Autodesk Inventor part; units mm, degrees
ref_plane "YZ Plane" through (0, 0, 0) normal (1, 0, 0) x (0, 1, 0)
ref_plane "XZ Plane" through (0, 0, 0) normal (0, 1, 0) x (-1, 0, 0)
ref_plane "XY Plane" through (0, 0, 0) normal (0, 0, 1) x (1, 0, 0)
sketch "Sketch1" plane through (0, 0, 0) normal (0, 0, 1) x (1, 0, 0)
  arc A0 (12.6748, 0.8001) -> (12.6748, -0.8001) centre (0, 0) ccw
  line L0 (-14.732, 25.4) -> (25.4, 25.4)
  line L1 (8.89, -14.732) -> (-8.382, -14.732)
  line L2 (-14.732, -8.382) -> (-14.732, 25.4)
  line L3 (-14.732, -8.382) -> (-8.382, -14.732)
  line L4 (8.89, -14.732) -> (15.24, -8.382)
  line L5 (15.24, -8.382) -> (25.4, -8.382)
  line L6 (-22.7584, 0) -> (33.4264, 0) construction
  line L7 (0, -22.7584) -> (0, 33.4264) construction
  line L8 (12.6748, 0.8001) -> (25.4, 0.8001)
  line L9 (12.6748, -0.8001) -> (25.4, -0.8001)
  line L10 (25.4, 25.4) -> (25.4, 0.8001)
  line L11 (25.4, -0.8001) -> (25.4, -8.382)
  dimension "d0" = 25.4
  dimension "d1" = 14.732
  dimension "d2" = 14.732
  dimension "d4" = 25.4
  dimension "d9" = 1.6002
  dimension "d11" = 45
  dimension "d12" = 25.4
  dimension "d14" = 8.89
  dimension "d15" = 15.24
  dimension "d49" = 45
extrude "Extrusion1" add sketch "Sketch1" along normal blind 12.7
sketch "Sketch2" plane through (0, 0, 12.7) normal (0, 0, 1) x (1, 0, 0)
  line L0 (-14.732, -8.382) -> (-14.732, 25.4)
  line L1 (-14.732, 25.4) -> (25.4, 25.4)
  line L2 (25.4, 25.4) -> (25.4, 0.8001)
  line L3 (-22.7584, 0) -> (33.4264, 0) construction
  line L4 (0, -22.7584) -> (0, 33.4264) construction
  line L5 (-11.557, 25.4) -> (22.225, 25.4)
  line L6 (22.225, 25.4) -> (22.225, 15.875)
  line L7 (19.05, 15.875) -> (-8.382, 15.875)
  line L8 (-11.557, 15.875) -> (-11.557, 25.4)
  arc A0 (-11.557, 15.875) -> (-8.382, 15.875) centre (-9.9695, 15.875) ccw
  arc A1 (19.05, 15.875) -> (22.225, 15.875) centre (20.6375, 15.875) ccw
  point P0 (0, 0)
  dimension "d16" = 3.175
  dimension "d17" = 3.175
  dimension "d18" = 9.525
  dimension "d19" = 3.175
extrude "Extrusion2" cut sketch "Sketch2" against normal blind 5.08
sketch "Sketch3" plane through (0, 0, 7.62) normal (0, 0, 1) x (1, 0, 0)
  line L0 (-11.557, 25.4) -> (22.225, 25.4)
  line L1 (-8.382, 15.875) -> (19.05, 15.875)
  line L2 (-5.207, 25.4) -> (15.875, 25.4)
  line L3 (15.875, 25.4) -> (15.875, 17.4752)
  line L4 (14.2748, 15.875) -> (-3.6068, 15.875)
  line L5 (-5.207, 17.4752) -> (-5.207, 25.4)
  arc A0 (-5.207, 17.4752) -> (-3.6068, 15.875) centre (-3.6068, 17.4752) ccw
  arc A1 (14.2748, 15.875) -> (15.875, 17.4752) centre (14.2748, 17.4752) ccw
  line L6 (5.334, 25.4) -> (5.334, 15.875) construction
  point P0 (0, 0)
  point P1 (15.875, 15.875)
  dimension "d22" = 1.6002
  dimension "d24" = 6.35
extrude "Extrusion3" cut sketch "Sketch3" against normal through all
sketch "Sketch4" plane through (0, 0, 7.62) normal (0, 0, 1) x (1, 0, 0)
  line L0 (22.225, 25.4) -> (22.225, 15.875)
  line L1 (-11.557, 25.4) -> (-11.557, 15.875)
  line L2 (-11.557, 20.6375) -> (22.225, 20.6375) construction
  line L3 (5.334, 29.021) -> (5.334, 12.254) construction
  point P0 (0, 0)
  point P1 (-7.366, 20.6375)
  point P2 (18.034, 20.6375)
  point P3 (23.8317, 40.0005)
  point P4 (5.334, 20.6375)
  dimension "d27" = 25.4
hole "Hole1" at (-7.366, 20.6375, 7.62) at (18.034, 20.6375, 7.62) at (23.8317, 40.0005, 7.62) direction (0, 0, -1) diameter 1.7018 end through all
sketch "Sketch5" plane through (15.24, -8.382, 0) normal (0, -1, 0) x (1, 0, 0)
  line L0 (10.16, 12.7) -> (0, 12.7)
  line L1 (0, 0) -> (0, 12.7)
  line L2 (10.16, 0) -> (0, 0)
  line L3 (10.16, 0) -> (10.16, 12.7)
  line L4 (5.08, 12.7) -> (5.08, 0) construction
  point P0 (-15.24, 0)
  point P1 (5.08, 6.35)
hole "Hole2" at (20.32, -8.382, 6.35) direction (0, 1, 0) diameter 4.4958 end up to surface counterbore diameter 7.9502 counterbore depth 4.1656
sketch "Sketch6" plane through (12.6748, 0.8001, 0) normal (0, -1, 0) x (1, 0, 0)
  circle A0 centre (7.6452, 6.35) radius 2.2479
  point P0 (-12.6748, 0)
hole "Hole3" at (20.32, 0.8001, 6.35) direction (0, 1, 0) diameter 3.302 depth 10.16 tip angle 118
fillet "Fillet1" radius 3.175 1 edges at (15.24, -8.382, 6.35)
equation "\"d1\" = d2"
equation "\"d14\" = d13"
equation "\"d17\" = d16"
properties part number "J002637" material "ALUMINUM, 6061-T651"
The listing builds one solid part. Answer for the finished solid, in the listing's coordinates (mm). A direction names the side the tool comes from. Coordinates: 2 decimals unless noted, no trailing zeros. Write each loop counter-clockwise with the first axis right and the second up, starting at its lowest first coordinate (ties: lowest second). Pieces come first, ordered by that corner, then holes. Notation, with made-up numbers: M 57.25,70.5 L 61.25,70.5 A21 ccw 61.25,80.5 Z; hole C 58.5,-13.5 d6. An arc over 180 degrees is marked long. Use a Markdown table: item, result. Add a question column.
1. Section B-B (y = 18.5) is taken. Give the vertices of the cut face in (x, z) (3 decimals), plus the area to 3 significant figures.
2. Which of the six approach directions +Z, -Z, +X, -X, +Y, -Y give full straight-line access (tool end or side, diameter ignored) to faces 4 (the cylindrical face through (24.2, -6.27, 7.21)), 5 (the flat face through (-14.732, 8, 6)), 6 (the flat face through (15.875, 21, 4)), 7 (the cylindrical face through (20.603, 14.288, 10.196))?
3. For a pull along Y with two mould halves and no side action, classify faces 1 (the flat face through (18, 0.8, 6)), 2 (the flat face through (11.57, -12.05, 6.26)), 3 (the cylindrical face through (19.204, 5.951, 7.567)) as +Y half, -Y half, draft (parallel to the pull), parting line (faces both ways), or undercut.
4. Given P1, Ø6.5, axis at x = 21.5, z = 5, coming from the -Y side; P2, Ø4, axis at x = 20.5, z = 7.5, coming from the -Y side; P3, Ø4, axis at x = -9, y = 19, coming from the +Z side, each flat-ended and moving along its own axis, determine where each tip first touches the part or whether it passes through.
5. Section A-A (x = 0) is taken. Give the vertices of the cut face in (y, z) (3 decimals), plus the area to 3 significant figures.
6. Section C-C (y = 5.5) is taken. Give the vertices of the cut face in (x, z), plus the area to 3 significant figures.
7. Straight lines are drawn through the part: line 1 along Y through (x, z) = (18, 5.25); line 2 along Z through (x, y) = (20.32, -7.45); line 3 along Y through (x, z) = (-0.5, 9) (3 decimals). For each, find the intervals that lie inside material, in ascending order. Write a range as [from, to].
Data:
| question | item | result |
|---|---|---|
| 1 | outline | M -14.732,0 L -5.207,0 L -5.207,7.62 L -11.557,7.62 L -11.557,12.7 L -14.732,12.7 Z; M 15.875,0 L 25.4,0 L 25.4,12.7 L 22.225,12.7 L 22.225,7.62 L 15.875,7.62 Z |
| 1 | area | 177 mm2 |
| 2 | face 4 | -Y |
| 2 | face 5 | +Z, -Z, -X, +Y, -Y |
| 2 | face 6 | +Z, -Z, +Y |
| 2 | face 7 | +Z, +Y |
| 3 | face 1 | undercut |
| 3 | face 2 | -Y half |
| 3 | face 3 | draft |
| 4 | P1 | stops at y = -8.38 |
| 4 | P2 | stops at y = -4.22 |
| 4 | P3 | stops at z = 7.62 |
| 5 | outline | M -14.732,0 L -12.7,0 L -12.7,12.7 L -14.732,12.7 Z; M 12.7,0 L 15.875,0 L 15.875,12.7 L 12.7,12.7 Z |
| 5 | area | 66.1 mm2 |
| 6 | outline | M -14.73,0 L -11.45,0 L -11.45,12.7 L -14.73,12.7 Z; M 11.45,0 L 25.4,0 L 25.4,12.7 L 11.45,12.7 Z; hole C 20.32,6.35 d3.3 |
| 6 | area | 210 mm2 |
| 7 | line 1 | y = [-4.22, -0.8], [0.8, 19.79], [21.49, 25.4] |
| 7 | line 2 | z = [0, 2.37], [10.33, 12.7] |
| 7 | line 3 | y = [-14.732, -12.69], [12.69, 15.875] |
